For this review, take the finished solid that the model builds, in its own axes (mm). Give positions to 0.01 mm unless a question says otherwise; leave off trailing zeros. Loops run counter-clockwise (first coordinate to the right, second up) from the corner with the lowest first, then second, coordinate; pieces in that order, holes last. Notation, with made-up numbers: M -7,86 L 2,86 A15 cw 2,113 Z; hole C -0.75,40 d7. An arc over 180 degrees is marked long. Use CSV: the item, a comma, the result in double quotes. Start each with the question number.
1. Take a section at A-A, the plane y = 44. Write out the cut boundary in (x, z), and give its area (3 significant figures).
2. Insertion check: P1, Ø2.5, axis at x = 0, z = 0, coming from the +Y side; P2, Ø4, axis at x = 1.5, y = -83.5, coming from the +Z side; P3, Ø3, axis at x = -2, z = 0, coming from the +Y side. Each pin has a flat end and moves straight along its axis. Give the tip position at first contact, or say it passes through.
3. To check wall thickness, follow line 1 (X direction, y = 106.5, z = 0); line 2 (X direction, y = 103.5, z = 0). State the ranges of each line that lie inside material, in increasing order. Write a range as [from, to].
from build123d import *

# Parameters (mm, degrees)
SKETCH_1_R      = 6
EXTRUDE_1_DEPTH = 115
SKETCH_2_W      = 1.5
SKETCH_2_H      = 210
CHAMFER_1_SIZE  = 1.5


with BuildPart() as part:
    # 草图1 → 凸台-拉伸1 (new, symmetric)
    with BuildSketch(Plane(origin=(0, 0, 0), x_dir=(1, 0, 0), z_dir=(0, 1, 0))):
        with Locations(Location((0, 0, 0), (0, 0, 270))):
            Circle(SKETCH_1_R)
    extrude(amount=EXTRUDE_1_DEPTH, both=True)

    # 草图2 → 切除-旋转1 (revolve, cut)
    with BuildSketch(Plane.XY, mode=Mode.PRIVATE) as cut_revolve_1_sk:
        with Locations((5.25, 0)):
            Rectangle(SKETCH_2_W, SKETCH_2_H)
    revolve(cut_revolve_1_sk.sketch.rotate(Axis((0, 115, 0), (0, -1, 0)), 90), axis=Axis((0, 115, 0), (0, -1, 0)), mode=Mode.SUBTRACT)

    # 倒角1
    chamfer_1_edges = [part.edges().sort_by_distance(p)[0] for p in [
        (0, 105, -4.5),
        (0, -105, -4.5),
    ]]
    chamfer(chamfer_1_edges, length=CHAMFER_1_SIZE - 0.0001)  # a hair under: the kernel refuses the full size

    # 草图3 → M5 螺纹孔1 (revolve, cut)
    with BuildSketch(Plane(origin=(0, -115, 0), x_dir=(0, 0, -1), z_dir=(1, 0, 0))):
        Polygon((0, 0), (0, 18.6618073), (2.1, 17.4), (2.1, 0), align=None)
    hole_wizard_m5_1 = revolve(axis=Axis((0, -121.35, 0), (0, 1, 0)), mode=Mode.SUBTRACT)

    # 镜向1: M5 螺纹孔1 across plane
    add(hole_wizard_m5_1.mirror(Plane.ZX), mode=Mode.SUBTRACT)


solid = part.part
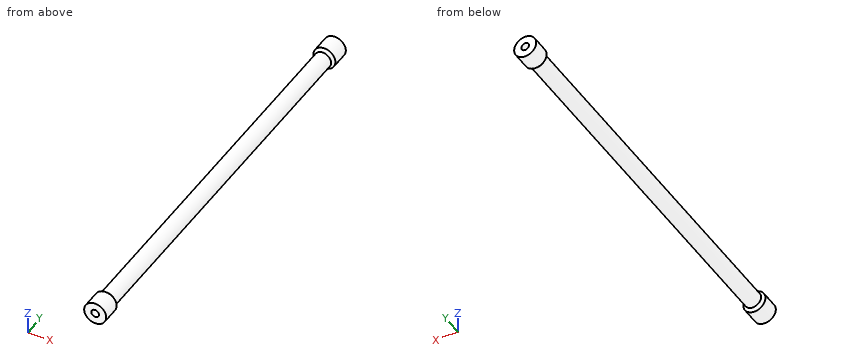
Result set:
1,outline,"C 0,0 d9"
1,area,"63.6 mm2"
2,P1,"y = 97.09"
2,P2,"z = 4.5"
2,P3,"y = 115"
3,line 1,"[-6, -2.1], [2.1, 6]"
3,line 2,"[-4.5, -2.1], [2.1, 4.5]"
